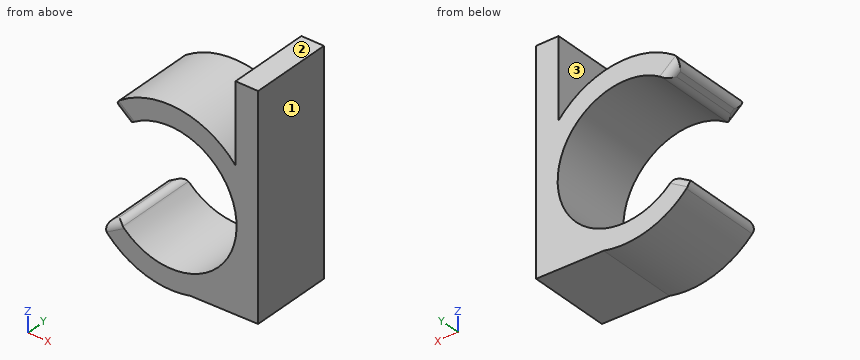
```python
from build123d import *

# Parameters (mm, degrees)
PAD_DEPTH   = 11
FILLET_R    = 1
FILLET001_R = 1


with BuildPart() as part:
    # Sketch → Pad (new body)
    with BuildSketch(Plane.XZ):
        with BuildLine():
            Line((0, 0), (0, 25))
            Line((0, 25), (-3, 25))
            Line((-3, 25), (-3, 14.5))
            ThreePointArc((-3, 14.5), (-10.968465, 18.475561), (-19.386255, 15.569992))
            Line((-17.306046, 13.862505), (-19.386255, 15.569992))
            ThreePointArc((-18.539906, 1.362505), (-2.9106, 6.130653), (-17.306046, 13.862505))
            Line((-18.539906, 1.362505), (-20.841942, 0))
            ThreePointArc((-20.841942, 0), (-15.540935, -3.845903), (-9, -4.174237))
            Line((-9, -4.174237), (0, -4))
            Line((0, 0), (0, -4))
        make_face()
    extrude(amount=PAD_DEPTH)

    # Fillet
    fillet_edges = [part.edges().sort_by_distance(p)[0] for p in [
        (-18.539906, -5.5, 1.362505),
        (-20.841942, -5.5, 0),
        (-19.690924, 0, 0.681253),
        (-19.690924, -11, 0.681253),
    ]]
    fillet(fillet_edges, radius=FILLET_R)

    # Fillet001
    fillet001_edges = [part.edges().sort_by_distance(p)[0] for p in [
        (-17.306046, -5.5, 13.862505),
        (-19.386255, -5.5, 15.569992),
        (-18.346151, 0, 14.716249),
        (-18.346151, -11, 14.716249),
    ]]
    fillet(fillet001_edges, radius=FILLET001_R)


solid = part.part
```
Source: CAD feature listing. Evaluate the final solid. Frame: model axes, mm. Face numbers are marked on the shaded views. Round coordinates to 2 decimals unless told otherwise and drop trailing zeros. Write each loop counter-clockwise with the first axis right and the second up, starting at its lowest first coordinate (ties: lowest second). Pieces come first, ordered by that corner, then holes. Notation, with made-up numbers: M 56,37.5 L 94,37.5 A8 cw 94,51.5 Z; hole C 1,-35.5 d2. An arc over 180 degrees is marked long. Answer as a JSON object with one key per item and string values. Group by question number.
(1) Mould query, pull axis X, two halves, no side actions, for the marked faces 1, 2 and 3. Classes: +X half, -X half, draft (parallel to the pull), parting line (faces both ways), or undercut.
(2) Section query A-A on x = -5.25. Output: boundary loops of the cut face in (y, z), then the cut area to 3 significant figures.
(3) Ray query, line 1 (X direction, y = -6.5, z = 7); line 2 (Z direction, x = -8.5, y = -5.5); line 3 (Z direction, x = -12.5, y = -2.25). Return the intervals inside material, ascending. Write a range as [from, to].
(4) First-contact query: pin 1 (5 mm diameter, centred on x = -18, y = -9.5, fed in from -Z); pin 2 (2 mm diameter, centred on x = -17.5, y = -4, fed in from +Z); pin 3 (5 mm diameter, centred on y = -6, z = 18.5, fed in from -X); pin 4 (1 mm diameter, centred on y = -8, z = 13, fed in from +X). Flat tips, straight axial feed; report the tip coordinate or a pass-through.
(5) Section query C-C on x = -15.5. Output: boundary loops of the cut face in (y, z).
(6) Section query B-B on y = -5. Output: boundary loops of the cut face in (x, z).
(7) Section query D-D on z = 7. Output: boundary loops of the cut face in (x, y).
Computed values:
{
 "1": {"face 1": "+X half", "face 2": "draft", "face 3": "undercut"},
 "2": {"outline": "M -11,-4.1 L 0,-4.1 L 0,0.96 L -11,0.96 Z; M -11,13.04 L 0,13.04 L 0,16.51 L -11,16.51 Z", "area": "93.8 mm^2"},
 "3": {"line 1": "[-2.87, 0]", "line 2": "[-4.16, -1.24], [15.24, 18.04]", "line 3": "[-4.47, -1.82], [15.82, 18.47]"},
 "4": {"pin 1": "z = -3.86", "pin 2": "z = 17.46", "pin 3": "x = -18.7", "pin 4": "x = 0"},
 "5": {"outline": "M -11,-3.86 L 0,-3.86 L 0,-1 L -11,-1 Z; M -11,15 L 0,15 L 0,17.86 L -11,17.86 Z"},
 "6": {"outline": "M -20.03,-0.95 A11.5 ccw -9,-4.17 L 0,-4 L 0,25 L -3,25 L -3,14.5 A11.5 ccw -18.38,16.38 A1 ccw -18.43,14.79 L -17.91,14.36 A1 ccw -16.71,14.31 A8.85 cw long -18.02,0.79 A1 ccw -19.24,0.95 L -19.82,0.61 A1 ccw Z"},
 "7": {"outline": "M -2.87,-11 L 0,-11 L 0,0 L -2.87,0 Z"}
}
